from build123d import *

# Parameters (mm, degrees)
F0_W     = 50.8
F0_H     = 25.4
F1_DEPTH = 254
F2_R     = 2.5527
F3_DEPTH = 25.4
F4_W     = 44.45
F4_H     = 19.05
F5_DEPTH = 254


with BuildPart() as f1:
    # F0 (on Top) → F1 (new body)
    with BuildSketch(Plane.XY):
        with Locations((-3.489516, 12.239771)):
            Rectangle(F0_W, F0_H)
    extrude(amount=F1_DEPTH)

    # F2 (on face) → F3 (cut)
    with BuildSketch(Plane.XZ.offset(0.460229)):
        with Locations((-16.189516, 241.3)):
            Circle(F2_R)
        with Locations((-16.189516, 215.9)):
            Circle(F2_R)
        with Locations((-16.189516, 190.5)):
            Circle(F2_R)
        with Locations((-16.189516, 165.1)):
            Circle(F2_R)
        with Locations((-16.189516, 139.7)):
            Circle(F2_R)
        with Locations((-16.189516, 114.3)):
            Circle(F2_R)
        with Locations((-16.189516, 88.9)):
            Circle(F2_R)
        with Locations((-16.189516, 63.5)):
            Circle(F2_R)
        with Locations((-16.189516, 38.1)):
            Circle(F2_R)
        with Locations((-16.189516, 12.7)):
            Circle(F2_R)
        with Locations((9.210484, 241.3)):
            Circle(F2_R)
        with Locations((9.210484, 215.9)):
            Circle(F2_R)
        with Locations((9.210484, 190.5)):
            Circle(F2_R)
        with Locations((9.210484, 165.1)):
            Circle(F2_R)
        with Locations((9.210484, 139.7)):
            Circle(F2_R)
        with Locations((9.210484, 114.3)):
            Circle(F2_R)
        with Locations((9.210484, 88.9)):
            Circle(F2_R)
        with Locations((9.210484, 63.5)):
            Circle(F2_R)
        with Locations((9.210484, 38.1)):
            Circle(F2_R)
        with Locations((9.210484, 12.7)):
            Circle(F2_R)
    extrude(amount=-F3_DEPTH, mode=Mode.SUBTRACT)

    # F4 (on face) → F5 (cut)
    with BuildSketch(Plane(origin=(0, 0, 0), x_dir=(1, 0, 0), z_dir=(0, 0, -1))):
        with Locations((-3.489516, -12.239771)):
            Rectangle(F4_W, F4_H)
    extrude(amount=-F5_DEPTH, mode=Mode.SUBTRACT)


solid = f1.part
Can you work these out from the model? Positions are in its coordinate system, mm. A direction names the side the tool comes from. Round coordinates to 2 decimals unless told otherwise and drop trailing zeros. Order: outer loops, then holes, each group sorted by start corner. A loop starts at its lowest first (then second) coordinate and runs counter-clockwise, first axis right, second up. Notation, with made-up numbers: M 66.5,34 L 104.5,34 A19 cw 104.5,62 Z; hole C 43,58 d7. An arc over 180 degrees is marked long. Use a Markdown table: item, result.
1) Imagine slicing it at B-B (x = -7). List the corners of the cut face in (y, z) for me, then the cut area to 3 significant figures.
Geometry says:
| item | result |
|---|---|
| outline | M -0.46,0 L 2.71,0 L 2.71,254 L -0.46,254 Z; M 21.76,0 L 24.94,0 L 24.94,254 L 21.76,254 Z |
| area | 1,610 mm² |
2) If we mould it in two halves opening along X, with no side actions, what happens to faces 3 (the face through (-4, -0.46, 125)), 4 (the face through (-16.7, 1.1, 213.4))? For each: +X half, -X half, draft (parallel to the pull), parting line (faces both ways), or undercut.
Geometry says:
| item | result |
|---|---|
| face 3 | draft |
| face 4 | undercut |
3) I'm going to push a flat-ended pin straight in: P1, Ø4.5, axis at x = 9.21, z = 63.5, coming from the +Y side. Where does the tip first touch, or does it pass through?
Geometry says:
| item | result |
|---|---|
| P1 | passes through |
4) On a 3-axis mill with a long thin cutter (end or side, diameter ignored), from which of +Z, -Z, +X, -X, +Y, -Y can I reach the whole of each face in a straight line? I mean faces 1 (the face through (-16.7, 1.1, 188)), 2 (the face through (-4, 2.715, 125)). Say none if no direction works.
Geometry says:
| item | result |
|---|---|
| face 1 | +Y, -Y |
| face 2 | +Z, -Z |
5) If I drill on line 1 along Y through (x, z) = (7.5, 183); line 2 along X through (y, z) = (10.25, 209), over which ranges is the centre line in solid material (lowest first)?
Geometry says:
| item | result |
|---|---|
| line 1 | y = -0.46 to 2.71, 21.76 to 24.94 |
| line 2 | x = -28.89 to -25.71, 18.74 to 21.91 |
6) Imagine slicing it at A-A (z = 12.7). List the corners of the cut face in (x, y) for me, then the cut area to 3 significant figures.
Geometry says:
| item | result |
|---|---|
| outline | M -28.89,-0.46 L -18.74,-0.46 L -18.74,2.71 L -25.71,2.71 L -25.71,21.76 L -18.74,21.76 L -18.74,24.94 L -28.89,24.94 Z; M -13.64,-0.46 L 6.66,-0.46 L 6.66,2.71 L -13.64,2.71 Z; M -13.64,21.76 L 6.66,21.76 L 6.66,24.94 L -13.64,24.94 Z; M 11.76,-0.46 L 21.91,-0.46 L 21.91,24.94 L 11.76,24.94 L 11.76,21.76 L 18.74,21.76 L 18.74,2.71 L 11.76,2.71 Z |
| area | 379 mm² |
7) Imagine slicing it at C-C (y = 10.5). List the corners of the cut face in (x, z) for me, then the cut area to 3 significant figures.
Geometry says:
| item | result |
|---|---|
| outline | M -28.89,0 L -25.71,0 L -25.71,254 L -28.89,254 Z; M 18.74,0 L 21.91,0 L 21.91,254 L 18.74,254 Z |
| area | 1,610 mm² |
